```python
from build123d import *

# Parameters (mm, degrees)
SKETCH1_W                      = 65
SKETCH1_H                      = 8.5
BOSS_EXTRUDE1_DEPTH            = 120
F_6_0MM_DOWEL_HOLE1_AT_2_COUNT = 2
F_6_0MM_DOWEL_HOLE1_AT_2_PITCH = 24.5
F_6_0MM_DOWEL_HOLE1_AT_3_COUNT = 2
F_6_0MM_DOWEL_HOLE1_AT_3_PITCH = 49
F_6_0MM_DOWEL_HOLE2_AT_2_COUNT = 2
F_6_0MM_DOWEL_HOLE2_AT_2_PITCH = 100
CUT_EXTRUDE1_DEPTH             = 9.5
F_3_0MM_DOWEL_HOLE1_D          = 3.5
CUT_EXTRUDE2_DEPTH             = 9.5
FILLET1_R                      = 6


with BuildPart() as part:
    # Sketch1 → Boss-Extrude1 (new body)
    with BuildSketch(Plane(origin=(0, 0, 0), x_dir=(0, 0, -1), z_dir=(1, 0, 0))):
        Rectangle(SKETCH1_W, SKETCH1_H)
    extrude(amount=BOSS_EXTRUDE1_DEPTH)

    # Sketch3 → Ø6.0mm Dowel Hole1 (revolve, cut)
    with BuildSketch(Plane(origin=(120, 0, 24.5), x_dir=(0, 0, -1), z_dir=(0, 1, 0))):
        Polygon((0, 0), (0, 11.802581857), (3, 10), (3, 0), align=None)
    f_6_0mm_dowel_hole1 = revolve(axis=Axis((126.35, 0, 24.5), (-1, 0, 0)), mode=Mode.SUBTRACT)

    # Ø6.0mm Dowel Hole1 at 2: Ø6.0mm Dowel Hole1 ×2
    with Locations(*[(0, 0, -i * F_6_0MM_DOWEL_HOLE1_AT_2_PITCH) for i in range(1, F_6_0MM_DOWEL_HOLE1_AT_2_COUNT)]):
        add(f_6_0mm_dowel_hole1, mode=Mode.SUBTRACT)

    # Ø6.0mm Dowel Hole1 at 3: Ø6.0mm Dowel Hole1 ×2
    with Locations(*[(0, 0, -i * F_6_0MM_DOWEL_HOLE1_AT_3_PITCH) for i in range(1, F_6_0MM_DOWEL_HOLE1_AT_3_COUNT)]):
        add(f_6_0mm_dowel_hole1, mode=Mode.SUBTRACT)

    # Mirror1: Ø6.0mm Dowel Hole1 across plane
    add(f_6_0mm_dowel_hole1.mirror(Plane(origin=(60, 0, 0), x_dir=(0, 0, 1), z_dir=(1, 0, 0))), mode=Mode.SUBTRACT)

    # Mirror1 copy 1 sketch → Mirror1 copy 1 (revolve, cut)
    with BuildSketch(Plane(origin=(0, 0, 0), x_dir=(0, 0, -1), z_dir=(0, 1, 0))):
        Polygon((0, 0), (0, -11.802581857), (3, -10), (3, 0), align=None)
    revolve(axis=Axis((-6.35, 0, 0), (-1, 0, 0)), mode=Mode.SUBTRACT)

    # Mirror1 copy 2 sketch → Mirror1 copy 2 (revolve, cut)
    with BuildSketch(Plane(origin=(0, 0, -24.5), x_dir=(0, 0, -1), z_dir=(0, 1, 0))):
        Polygon((0, 0), (0, -11.802581857), (3, -10), (3, 0), align=None)
    revolve(axis=Axis((-6.35, 0, -24.5), (-1, 0, 0)), mode=Mode.SUBTRACT)

    # Sketch5 → Ø6.0mm Dowel Hole2 (revolve, cut)
    with BuildSketch(Plane(origin=(110, 0, -32.5), x_dir=(0, 1, 0), z_dir=(1, 0, 0))):
        Polygon((0, 0), (0, 9.802581857), (3, 8), (3, 0), align=None)
    f_6_0mm_dowel_hole2 = revolve(axis=Axis((110, 0, -38.85), (0, 0, 1)), mode=Mode.SUBTRACT)

    # Ø6.0mm Dowel Hole2 at 2: Ø6.0mm Dowel Hole2 ×2
    with Locations(*[(-i * F_6_0MM_DOWEL_HOLE2_AT_2_PITCH, 0, 0) for i in range(1, F_6_0MM_DOWEL_HOLE2_AT_2_COUNT)]):
        add(f_6_0mm_dowel_hole2, mode=Mode.SUBTRACT)

    # Mirror2: Ø6.0mm Dowel Hole2 across plane
    add(f_6_0mm_dowel_hole2.mirror(Plane.XY), mode=Mode.SUBTRACT)

    # Mirror2 copy 1 sketch → Mirror2 copy 1 (revolve, cut)
    with BuildSketch(Plane(origin=(10, 0, 32.5), x_dir=(0, 1, 0), z_dir=(1, 0, 0))):
        Polygon((0, 0), (0, -9.802581857), (3, -8), (3, 0), align=None)
    revolve(axis=Axis((10, 0, 38.85), (0, 0, 1)), mode=Mode.SUBTRACT)

    # Sketch6 → Cut-Extrude1 (cut, through all)
    with BuildSketch(Plane(origin=(0, 4.25, 0), x_dir=(1, 0, 0), z_dir=(0, 1, 0))):
        with BuildLine():
            Line((80, -7), (80, 7))
            ThreePointArc((80, 7), (86, 13), (92, 7))
            Line((92, 7), (92, -7))
            ThreePointArc((92, -7), (86, -13), (80, -7))
        make_face()
    cut_extrude1 = extrude(amount=-CUT_EXTRUDE1_DEPTH, mode=Mode.SUBTRACT)

    # Mirror3: Cut-Extrude1 across plane
    add(cut_extrude1.mirror(Plane(origin=(60, 0, 0), x_dir=(0, 0, 1), z_dir=(1, 0, 0))), mode=Mode.SUBTRACT)

    # Ø3.0mm Dowel Hole1 (through all)
    with Locations(Plane(origin=(0, 4.25, 0), x_dir=(1, 0, 0), z_dir=(0, 1, 0))):
        with Locations((87, -17), (87, 17), (33, 17), (33, -17), (100, -24.5), (60, -24.5), (20, -24.5), (100, 24.5), (60, 24.5), (20, 24.5)):
            Hole(F_3_0MM_DOWEL_HOLE1_D / 2)

    # Sketch10 → Cut-Extrude2 (cut, through all)
    with BuildSketch(Plane.XZ.offset(4.25)):
        with BuildLine():
            ThreePointArc((34, 13), (38.242640687, 11.242640687), (40, 7))
            Line((40, 7), (40, 21.5))
            Line((40, 21.5), (34, 13))
        make_face()
        Polygon((40, -7), (40, -21.5), (80, -21.5), (80, -7), (80, 7), (80, 21.5), (40, 21.5), (40, 7), align=None)
        with BuildLine():
            Line((34, -13), (40, -21.5))
            Line((40, -21.5), (40, -7))
            ThreePointArc((40, -7), (38.242640687, -11.242640687), (34, -13))
        make_face()
        with BuildLine():
            Line((80, 21.5), (80, 7))
            ThreePointArc((80, 7), (81.757359313, 11.242640687), (86, 13))
            Line((86, 13), (80, 21.5))
        make_face()
        with BuildLine():
            Line((80, -7), (80, -21.5))
            Line((80, -21.5), (86, -13))
            ThreePointArc((86, -13), (81.757359313, -11.242640687), (80, -7))
        make_face()
    extrude(amount=-CUT_EXTRUDE2_DEPTH, mode=Mode.SUBTRACT)

    # Fillet1
    fillet1_edges = [part.edges().sort_by_distance(p)[0] for p in [
        (34, 0, 13),
        (40, 0, 21.5),
        (80, 0, 21.5),
        (86, 0, 13),
        (86, 0, -13),
        (80, 0, -21.5),
        (40, 0, -21.5),
        (34, 0, -13),
    ]]
    fillet(fillet1_edges, radius=FILLET1_R)


solid = part.part
```
For this review, take the finished solid that the model builds, in its own axes (mm). A direction names the side the tool comes from. Round coordinates to 2 decimals unless told otherwise and drop trailing zeros. Write each loop counter-clockwise with the first axis right and the second up, starting at its lowest first coordinate (ties: lowest second). Pieces come first, ordered by that corner, then holes. Notation, with made-up numbers: (-36, -20) - (-1, -20) arc R18 cw to (-1, 8) - close; hole circle Ø8 at (64, -22). An arc over 180 degrees is marked (long way). Use CSV: the item, a comma, the result in double quotes.
1) Add section B-B on z = 11. Write out the cut boundary in (x, y).
Conclusion:
outline,"(0, -4.25) - (29.53, -4.25) - (29.53, 4.25) - (0, 4.25) - close; (90.47, -4.25) - (120, -4.25) - (120, 4.25) - (90.47, 4.25) - close"
2) Clearance check with flat-ended pins moving along their axes: pin 1 Ø3.5 at (x, y) = (10, 0) entering from -Z; pin 2 Ø5 at (y, z) = (0, 0) entering from -X; pin 3 Ø2 at (x, z) = (20, -24.5) entering from +Y. State where each tip first meets the part, or that it passes through.
Conclusion:
pin 1,"stops at z = -23.75"
pin 2,"stops at x = 10.3"
pin 3,"passes through"
3) For faces 1 (the cylindrical face through (115.07, 1.15, -2.77)), 2 (the flat face through (36.84, -0.06, 17.02)), 3 (the cylindrical face through (107, 0, -29)), 4 (the cylindrical face through (12.93, -0.65, 28.56)), list the 3-axis set-ups (+Z, -Z, +X, -X, +Y, -Y) from which the entire face can be reached by the end or side of a thin tool; tool diameter is ignored.
Conclusion:
face 1,"+X"
face 2,"+Y, -Y"
face 3,"-Z"
face 4,"+Z"
4) Add section D-D on x = 79. Write out the cut boundary in (y, z).
Conclusion:
outline,"(-4.25, -32.5) - (4.25, -32.5) - (4.25, -21.12) - (-4.25, -21.12) - close; (-4.25, 21.12) - (4.25, 21.12) - (4.25, 32.5) - (-4.25, 32.5) - close"
5) Add section A-A on x = 60. Write out the cut boundary in (y, z), and give its area (4 significant figures).
Conclusion:
outline,"(-4.25, -32.5) - (4.25, -32.5) - (4.25, -26.25) - (-4.25, -26.25) - close; (-4.25, -22.75) - (4.25, -22.75) - (4.25, -21.5) - (-4.25, -21.5) - close; (-4.25, 21.5) - (4.25, 21.5) - (4.25, 22.75) - (-4.25, 22.75) - close; (-4.25, 26.25) - (4.25, 26.25) - (4.25, 32.5) - (-4.25, 32.5) - close"
area,"127.5 mm^2"
6) Add section C-C on x = 100. Write out the cut boundary in (y, z), and give its area (3 significant figures).
Conclusion:
outline,"(-4.25, -32.5) - (4.25, -32.5) - (4.25, -26.25) - (-4.25, -26.25) - close; (-4.25, -22.75) - (4.25, -22.75) - (4.25, 22.75) - (-4.25, 22.75) - close; (-4.25, 26.25) - (4.25, 26.25) - (4.25, 32.5) - (-4.25, 32.5) - close"
area,"493 mm^2"
7) Wall thickness on line 1 along Z through (x, y) = (3, 0); line 2 along Z through (x, y) = (60, -1); line 3 along X through (y, z) = (0, 30.5): over which ranges is each line inside the solid? List them lowest first. Write a range as from..to.
Conclusion:
line 1,"z = -32.5..-27.5, -21.5..-3, 3..21.5, 27.5..32.5"
line 2,"z = -32.5..-26.25, -22.75..-21.5, 21.5..22.75, 26.25..32.5"
line 3,"x = 0..7, 13..107, 113..120"
8) The part is to be moulded in two halves that separate along Z. For faces 5 (the flat face through (59, 0, -32.5)), 6 (the conical face through (108.341, 0.036, 23.695)), 7 (the flat face through (60, 0, 21.5)), say which applies: pulls with the +Z half, pulls with the -Z half, needs draft (parallel to the pull), parting line crosses it, or undercut.
Conclusion:
face 5,"pulls with the -Z half"
face 6,"pulls with the +Z half"
face 7,"undercut"
